from build123d import *

# Parameters (mm, degrees)
BOSS_EXTRUDE1_DEPTH = 3
FILLET1_R           = 5
CUT_EXTRUDE1_REACH  = 5
SKETCH2_R           = 1.5


with BuildPart() as part:
    # Sketch1 → Boss-Extrude1 (new body)
    with BuildSketch(Plane(origin=(0, 0, 0), x_dir=(1, 0, 0), z_dir=(0, 1, 0))):
        with BuildLine():
            Line((-68.408481347, 122.148596717), (-54.266345723, 108.006461093))
            ThreePointArc((-54.266345723, 108.006461093), (0, 127.583500889), (54.266345723, 108.006461093))
            Line((54.266345723, 108.006461093), (68.408481347, 122.148596717))
            ThreePointArc((68.408481347, 122.148596717), (0, 140), (-68.408481347, 122.148596717))
        make_face()
    extrude(amount=BOSS_EXTRUDE1_DEPTH)

    # Fillet1
    fillet1_edges = [part.edges().sort_by_distance(p)[0] for p in [
        (68.408481347, 1.5, -122.148596717),
        (54.266345723, 1.5, -108.006461093),
        (-54.266345723, 1.5, -108.006461093),
        (-68.408481347, 1.5, -122.148596717),
    ]]
    fillet(fillet1_edges, radius=FILLET1_R)

    # Sketch2 → Cut-Extrude1 (cut, up to next)
    with BuildSketch(Plane(origin=(0, 3, 0), x_dir=(1, 0, 0), z_dir=(0, 1, 0)), mode=Mode.PRIVATE) as cut_extrude1_sk1:
        with Locations((-50, 120)):
            Circle(SKETCH2_R)
    cut_extrude1_tool1 = extrude(cut_extrude1_sk1.sketch, amount=-CUT_EXTRUDE1_REACH, mode=Mode.PRIVATE) & part.part
    add(cut_extrude1_tool1.solids().sort_by_distance((-50, 3, -120))[0], mode=Mode.SUBTRACT)
    # Sketch2 → Cut-Extrude1 (cut, up to next)
    with BuildSketch(Plane(origin=(0, 3, 0), x_dir=(1, 0, 0), z_dir=(0, 1, 0)), mode=Mode.PRIVATE) as cut_extrude1_sk2:
        with Locations((50, 120)):
            Circle(SKETCH2_R)
    cut_extrude1_tool2 = extrude(cut_extrude1_sk2.sketch, amount=-CUT_EXTRUDE1_REACH, mode=Mode.PRIVATE) & part.part
    add(cut_extrude1_tool2.solids().sort_by_distance((50, 3, -120))[0], mode=Mode.SUBTRACT)


solid = part.part
Model file for the job. Use its own axes, mm. Give positions to 0.01 mm unless a question says otherwise; leave off trailing zeros. Write each loop counter-clockwise with the first axis right and the second up, starting at its lowest first coordinate (ties: lowest second). Pieces come first, ordered by that corner, then holes. Notation, with made-up numbers: M -14,9.5 L 44,9.5 A19 cw 44,31.5 Z; hole C -2,89 d6. An arc over 180 degrees is marked long. One line per item, written item: value. Start each with the question number.
Q1. Saw through at C-C, the plane x = 7.5. Write the cut outline in (y, z), plus the area to 3 significant figures.
Q2. Probe probe 1 along X at (y, z) = (1.4, -120); probe 2 along Z at (x, y) = (50, 1.95); probe 3 along Z at (x, y) = (-49, 0.9). List the from-to ranges inside material, lowest first. Write a range as [from, to].
Q3. Saw through at A-A, the plane z = -120. Write the cut outline in (x, y), plus the area to 3 significant figures.
Q4. Two-plate mould, pull along X, no slides. Class faces 1 (the flat face through (-60.555, 1.479, -114.295)), 2 (the cylindrical face through (54.18, 1.52, -109.69)), 3 (the cylindrical face through (0.904, 1.479, -139.997)): +X half, -X half, draft (parallel to the pull), parting line (faces both ways), or undercut.
Q5. Saw through at D-D, the plane z = -136. Write the cut outline in (x, y).
Q6. Drop a flat-ended pin along its axis: pin 1 Ø8 at (x, z) = (38, -135.5) entering from +Y. Give the stop position or say it passes through.
Q7. Saw through at B-B, the plane y = 0.6. Write the cut outline in (x, z).
Output values:
1. outline: M 0,-139.8 L 3,-139.8 L 3,-127.25 L 0,-127.25 Z
1. area: 37.6 mm²
2. probe 1: x = [-65, -51.5], [-48.5, -35.1], [35.1, 48.5], [51.5, 65]
2. probe 2: z = [-130.77, -121.5], [-118.5, -111.32]
2. probe 3: z = [-131.14, -121.12], [-118.88, -112.04]
3. outline: M -65,0 L -51.5,0 L -51.5,3 L -65,3 Z; M -48.5,0 L -35.1,0 L -35.1,3 L -48.5,3 Z; M 35.1,0 L 48.5,0 L 48.5,3 L 35.1,3 Z; M 51.5,0 L 65,0 L 65,3 L 51.5,3 Z
3. area: 161 mm²
4. face 1: -X half
4. face 2: undercut
4. face 3: parting line
5. outline: M -33.23,0 L 33.23,0 L 33.23,3 L -33.23,3 Z
6. pin 1: stops at y = 3
7. outline: M -63.62,-117.36 A5 ccw -62.31,-125.37 A140 ccw 62.31,-125.37 A5 ccw 63.62,-117.36 L 57.41,-111.15 A5 ccw 50.88,-110.68 A85 cw -50.88,-110.68 A5 ccw -57.41,-111.15 Z; hole C -50,-120 d3; hole C 50,-120 d3
